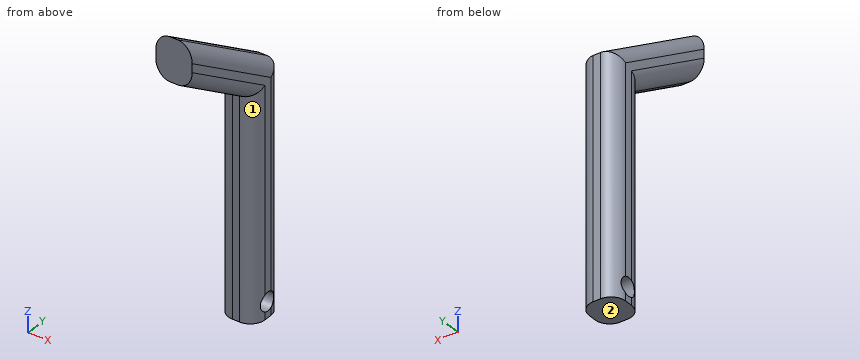
from build123d import *

# Parameters (mm, degrees)
F0_R         = 3.175
F1_DEPTH     = 12.7
F3_DEPTH     = 12.701
F4_T1_DEPTH  = 108.2499657273
F4_T3_DEPTH  = 76.2
F4_T8_DEPTH  = 101.5317029417
F4_T13_DEPTH = 101.5317029417
F4_T18_DEPTH = 60.7438000865
F4_T23_DEPTH = 60.7438000865
F4_T29_DEPTH = 101.5317029417
F4_T33_DEPTH = 60.7438000865
F4_T40_DEPTH = 101.5317029417
F4_T44_DEPTH = 60.7438000865


# Not quite as in the source:
# - a fillet or chamfer that OpenCascade refuses, or shapes differently, is made with other operations: its cross-section is extruded or revolved along the edge and cut away or added


with BuildPart() as f1:
    # F0 (on Right) → F1 (new body)
    with BuildSketch(Plane.YZ):
        Polygon((-12.9443686455, 18.7500342727), (0, 18.7500342727), (0, 101.6), (-42.5443466617, 129.3600174195), (-49.4843510166, 118.7239307541), (-12.9443686455, 94.8817372144), align=None)
        with Locations((-6.4721843228, 24.2384169251)):
            Circle(F0_R, mode=Mode.SUBTRACT)
    extrude(amount=F1_DEPTH)

    # F2 (on face) → F3 (cut, through all)
    with BuildSketch(Plane(origin=(0, 0, 0), x_dir=(0, -1, 0), z_dir=(-1, 0, 0))):
        Polygon((49.4843510166, 118.7239307541), (42.5443466617, 129.3600174195), (42.5443466617, 114.1956054441), align=None)
    extrude(amount=-F3_DEPTH, mode=Mode.SUBTRACT)

    # F4: fillet of radius 5.08 on 8 edges, made by hand

    # F4_s2 → F4_t1 (cut)
    with BuildSketch(Plane.XY.offset(6.0500342727)):
        with BuildLine():
            ThreePointArc((0, -5.08), (1.4878975516, -1.4878975516), (5.08, 0))
            Line((5.08, 0), (0, 0))
            Line((0, 0), (0, -5.08))
        make_face()
        with BuildLine():
            ThreePointArc((12.7, -5.08), (11.2121024484, -1.4878975516), (7.62, 0))
            Line((7.62, 0), (12.7, 0))
            Line((12.7, 0), (12.7, -5.08))
        make_face()
    extrude(amount=F4_T1_DEPTH, mode=Mode.SUBTRACT)

    # F4_s4 → F4_t3 (cut)
    with BuildSketch(Plane(origin=(0, -35.8612284696, 23.3993093117), x_dir=(1, 0, 0), z_dir=(0, -0.837487139, 0.5464570358))):
        with BuildLine():
            ThreePointArc((12.7, 80.0086933233), (11.2121024484, 83.6007957718), (7.62, 85.0886933233))
            Line((7.62, 85.0886933233), (12.7, 85.0886933233))
            Line((12.7, 85.0886933233), (12.7, 80.0086933233))
        make_face()
        with BuildLine():
            ThreePointArc((0, 80.0086933233), (1.4878975516, 83.6007957718), (5.08, 85.0886933233))
            Line((5.08, 85.0886933233), (0, 85.0886933233))
            Line((0, 85.0886933233), (0, 80.0086933233))
        make_face()
    extrude(amount=F4_T3_DEPTH, mode=Mode.SUBTRACT)


with BuildPart() as f4_tool6:
    # F4_s7 → F4_t8 (new body)
    with BuildSketch(Plane.XY.offset(107.5817372144)):
        with BuildLine():
            ThreePointArc((5.08, -12.9443686455), (1.4878975516, -11.456471094), (0, -7.8643686455))
            Line((0, -7.8643686455), (0, -12.9443686455))
            Line((0, -12.9443686455), (5.08, -12.9443686455))
        make_face()
    extrude(amount=-F4_T8_DEPTH)

    split(bisect_by=Plane(origin=(0, 39.5573107801, 60.624599668), x_dir=(1, 0, 0), z_dir=(0, -0.5464570358, -0.837487139)), keep=Keep.TOP)


with BuildPart() as f1_1:
    add(f1.part)

    # F4_t5: cut F4_tool6
    add(f4_tool6.part, mode=Mode.SUBTRACT)


with BuildPart() as f4_tool11:
    # F4_s12 → F4_t13 (new body)
    with BuildSketch(Plane.XY.offset(107.5817372144)):
        with BuildLine():
            ThreePointArc((7.62, -12.9443686455), (11.2121024484, -11.456471094), (12.7, -7.8643686455))
            Line((12.7, -7.8643686455), (12.7, -12.9443686455))
            Line((12.7, -12.9443686455), (7.62, -12.9443686455))
        make_face()
    extrude(amount=-F4_T13_DEPTH)

    split(bisect_by=Plane(origin=(0, 39.5573107801, 60.624599668), x_dir=(1, 0, 0), z_dir=(0, -0.5464570358, -0.837487139)), keep=Keep.TOP)


with BuildPart() as f1_2:
    add(f1_1.part)

    # F4_t10: cut F4_tool11
    add(f4_tool11.part, mode=Mode.SUBTRACT)


with BuildPart() as f4_tool16:
    # F4_s17 → F4_t18 (new body)
    with BuildSketch(Plane(origin=(0, -92.7377441072, 60.511010131), x_dir=(1, 0, 0), z_dir=(0, 0.837487139, -0.5464570358))):
        with BuildLine():
            ThreePointArc((7.62, -72.3886933233), (11.2121024484, -73.8765908749), (12.7, -77.4686933233))
            Line((12.7, -77.4686933233), (12.7, -72.3886933233))
            Line((12.7, -72.3886933233), (7.62, -72.3886933233))
        make_face()
    extrude(amount=F4_T18_DEPTH)

    split(bisect_by=Plane.XZ.offset(12.9443686455), keep=Keep.TOP)


with BuildPart() as f1_3:
    add(f1_2.part)

    # F4_t15: cut F4_tool16
    add(f4_tool16.part, mode=Mode.SUBTRACT)


with BuildPart() as f4_tool21:
    # F4_s22 → F4_t23 (new body)
    with BuildSketch(Plane(origin=(0, -92.7377441072, 60.511010131), x_dir=(1, 0, 0), z_dir=(0, 0.837487139, -0.5464570358))):
        with BuildLine():
            ThreePointArc((5.08, -72.3886933233), (1.4878975516, -73.8765908749), (0, -77.4686933233))
            Line((0, -77.4686933233), (0, -72.3886933233))
            Line((0, -72.3886933233), (5.08, -72.3886933233))
        make_face()
    extrude(amount=F4_T23_DEPTH)

    split(bisect_by=Plane.XZ.offset(12.9443686455), keep=Keep.TOP)


with BuildPart() as f1_4:
    add(f1_3.part)

    # F4_t20: cut F4_tool21
    add(f4_tool21.part, mode=Mode.SUBTRACT)


with BuildPart() as f4_tool27:
    # F4_s28 → F4_t29 (new body)
    with BuildSketch(Plane.XY.offset(107.5817372144)):
        with BuildLine():
            ThreePointArc((5.08, -12.9443686455), (1.4878975516, -11.456471094), (0, -7.8643686455))
            Line((0, -7.8643686455), (0, -12.9443686455))
            Line((0, -12.9443686455), (5.08, -12.9443686455))
        make_face()
    extrude(amount=-F4_T29_DEPTH)

    split(bisect_by=Plane(origin=(0, 39.5573107801, 60.624599668), x_dir=(1, 0, 0), z_dir=(0, 0.5464570358, 0.837487139)), keep=Keep.TOP)


with BuildPart() as f4_tool31:
    # F4_s32 → F4_t33 (new body)
    with BuildSketch(Plane(origin=(0, -92.7377441072, 60.511010131), x_dir=(1, 0, 0), z_dir=(0, 0.837487139, -0.5464570358))):
        with BuildLine():
            ThreePointArc((5.08, -72.3886933233), (1.4878975516, -73.8765908749), (0, -77.4686933233))
            Line((0, -77.4686933233), (0, -72.3886933233))
            Line((0, -72.3886933233), (5.08, -72.3886933233))
        make_face()
    extrude(amount=F4_T33_DEPTH)

    split(bisect_by=Plane.XZ.offset(12.9443686455), keep=Keep.BOTTOM)


with BuildPart() as f4_tool27_1:
    add(f4_tool27.part)

    # F4_t35: intersect F4_tool31
    add(f4_tool31.part, mode=Mode.INTERSECT)


with BuildPart() as f1_5:
    add(f1_4.part)

    # F4_t25: cut F4_tool27
    add(f4_tool27_1.part, mode=Mode.SUBTRACT)


with BuildPart() as f4_tool38:
    # F4_s39 → F4_t40 (new body)
    with BuildSketch(Plane.XY.offset(107.5817372144)):
        with BuildLine():
            ThreePointArc((7.62, -12.9443686455), (11.2121024484, -11.456471094), (12.7, -7.8643686455))
            Line((12.7, -7.8643686455), (12.7, -12.9443686455))
            Line((12.7, -12.9443686455), (7.62, -12.9443686455))
        make_face()
    extrude(amount=-F4_T40_DEPTH)

    split(bisect_by=Plane(origin=(0, 39.5573107801, 60.624599668), x_dir=(1, 0, 0), z_dir=(0, 0.5464570358, 0.837487139)), keep=Keep.TOP)


with BuildPart() as f4_tool42:
    # F4_s43 → F4_t44 (new body)
    with BuildSketch(Plane(origin=(0, -92.7377441072, 60.511010131), x_dir=(1, 0, 0), z_dir=(0, 0.837487139, -0.5464570358))):
        with BuildLine():
            ThreePointArc((7.62, -72.3886933233), (11.2121024484, -73.8765908749), (12.7, -77.4686933233))
            Line((12.7, -77.4686933233), (12.7, -72.3886933233))
            Line((12.7, -72.3886933233), (7.62, -72.3886933233))
        make_face()
    extrude(amount=F4_T44_DEPTH)

    split(bisect_by=Plane.XZ.offset(12.9443686455), keep=Keep.BOTTOM)


with BuildPart() as f4_tool38_1:
    add(f4_tool38.part)

    # F4_t46: intersect F4_tool42
    add(f4_tool42.part, mode=Mode.INTERSECT)


with BuildPart() as f1_6:
    add(f1_5.part)

    # F4_t36: cut F4_tool38
    add(f4_tool38_1.part, mode=Mode.SUBTRACT)


solid = f1_6.part
Verification items for the finished model (mm, model axes). Face numbers are marked on the shaded views. A direction names the side the tool comes from. Coordinates: 2 decimals unless noted, no trailing zeros. Order: outer loops, then holes, each group sorted by start corner. A loop starts at its lowest first (then second) coordinate and runs counter-clockwise, first axis right, second up. Notation, with made-up numbers: M 75.25,-16.5 L 113.25,-16.5 A20 ccw 113.25,2.5 Z; hole C 75,-11.5 d2. An arc over 180 degrees is marked long. One line per item, written item: value. Start each with the question number.
Item 1: Scan lines: probe 1 along Y at (x, z) = (6.75, 64); probe 2 along Z at (x, y) = (10, -7); probe 3 along Z at (x, y) = (4.75, -24.5). Record each from-to range of solid material in increasing order.
Item 2: Access from +Z, -Z, +X, -X, +Y, -Y to the whole of each face (thin tool, end or side, straight path). Record for the marked faces 1 and 2.
Item 3: Sectioned sample at C-C (x = 3.5). Enter the section's corners in (y, z) (3 decimals), then the cut area to 3 significant figures.
Item 4: Gauge pin test, flat ends, axial feed: pin 1 (5 mm diameter, centred on x = 8.5, y = -36, fed in from +Z); pin 2 (2 mm diameter, centred on x = 2.5, y = -31, fed in from -Z); pin 3 (3 mm diameter, centred on x = 10.5, z = 111, fed in from -Y). Record the tip position at first contact, or that the pin passes through.
Item 5: Sectioned sample at B-B (z = 91). Enter the section's corners in (x, y), then the cut area to 3 significant figures.
Conclusion:
1. probe 1: y = -12.94 to 0
1. probe 2: z = 18.75 to 21.11, 27.37 to 105.46
1. probe 3: z = 102.43 to 117.57
2. face 1: -Z, +X, -Y
2. face 2: -Z, +X, -X, +Y, -Y
3. outline: M -42.544,114.496 L -12.692,95.018 L -12.692,18.75 L -0.252,18.75 L -0.252,101.464 L -42.544,129.059 Z; hole C -6.472,24.238 d6.35
3. area: 1,480 mm^2
4. pin 1: stops at z = 126.67
4. pin 2: stops at z = 106.62
4. pin 3: stops at y = -38.78
5. outline: M 0,-7.86 A5.08 ccw 5.08,-12.94 L 7.62,-12.94 A5.08 ccw 12.7,-7.86 L 12.7,-5.08 A5.08 ccw 7.62,0 L 5.08,0 A5.08 ccw 0,-5.08 Z
5. area: 142 mm^2
